from build123d import *

# Parameters (mm, degrees)
F0_W     = 12.7
F0_H     = 6.35
F1_DEPTH = 6.35


with BuildPart() as f1:
    # F0 (on Top) → F1 (new body)
    with BuildSketch(Plane.XY):
        Polygon((12.7, 0), (0, 0), (0, -50.8), (12.7, -50.8), (38.1, -50.8), (50.8, -50.8), (50.8, 0), (38.1, 0), align=None)
        with Locations((6.35, -53.975)):
            Rectangle(F0_W, F0_H)
        with Locations((44.45, -53.975)):
            Rectangle(F0_W, F0_H)
        with Locations((6.35, 3.175)):
            Rectangle(F0_W, F0_H)
        with Locations((44.45, 3.175)):
            Rectangle(F0_W, F0_H)
    extrude(amount=F1_DEPTH)


solid = f1.part
Source: CAD feature listing. Evaluate the final solid. Frame: model axes, mm. A direction names the side the tool comes from. Round coordinates to 2 decimals unless told otherwise and drop trailing zeros. Loops run counter-clockwise (first coordinate to the right, second up) from the corner with the lowest first, then second, coordinate; pieces in that order, holes last.
Q1. Section B-B, the plane x = 33. Return loops of the section in (y, z), plus the area to 3 significant figures.
Q2. Access query for faces 4 (the face through (25, -50.8, 3)), 5 (the face through (44, -57.15, 3)), 6 (the face through (26, 0, 3)). Directions: +Z, -Z, +X, -X, +Y, -Y. A direction counts if a zero-diameter tool reaches every point of the face in a straight line with its end or side. Return the directions, or none.
Q3. Mould query, pull axis X, two halves, no side actions, for faces 1 (the face through (25, -25, 0)), 2 (the face through (50.8, -26, 3)), 3 (the face through (12.7, 3, 3)). Classes: pulls with the +X half, pulls with the -X half, needs draft (parallel to the pull), parting line crosses it, or undercut.
Q4. Section A-A, the plane z = 4.5. Return loops of the section in (x, y), plus the area to 3 significant figures.
Q5. Ray query, line 1 (X direction, y = 1, z = 5.5); line 2 (Y direction, x = 20.5, z = 1.5). Return the intervals inside material, ascending.
Solutions:
1. outline: (-50.8, 0) - (0, 0) - (0, 6.35) - (-50.8, 6.35) - close
1. area: 323 mm2
2. face 4: +Z, -Z, -Y
2. face 5: +Z, -Z, +X, -X, -Y
2. face 6: +Z, -Z, +Y
3. face 1: needs draft
3. face 2: pulls with the +X half
3. face 3: undercut
4. outline: (0, -57.15) - (12.7, -57.15) - (12.7, -50.8) - (38.1, -50.8) - (38.1, -57.15) - (50.8, -57.15) - (50.8, 6.35) - (38.1, 6.35) - (38.1, 0) - (12.7, 0) - (12.7, 6.35) - (0, 6.35) - close
4. area: 2,900 mm2
5. line 1: x = 0 to 12.7, 38.1 to 50.8
5. line 2: y = -50.8 to 0
